Can you work these out from the model? Positions are in its coordinate system, mm. A direction names the side the tool comes from. Give positions to 0.01 mm unless a question says otherwise; leave off trailing zeros. Write each loop counter-clockwise with the first axis right and the second up, starting at its lowest first coordinate (ties: lowest second). Pieces come first, ordered by that corner, then holes.
from build123d import *

# Parameters (mm, degrees)
SKETCH_1_W      = 30
SKETCH_1_H      = 15
SKETCH_1_R      = 1.75
EXTRUDE_1_DEPTH = 1.5
FILLET_1_R      = 5
EXTRUDE_2_DEPTH = 10


with BuildPart() as part:
    # 草图1 → 凸台-拉伸1 (new body)
    with BuildSketch(Plane(origin=(0, 0, 0), x_dir=(1, 0, 0), z_dir=(0, 1, 0))):
        Rectangle(SKETCH_1_W, SKETCH_1_H)
        with Locations(Location((-8.867330988, 0, 0), (0, 0, 270))):
            Circle(SKETCH_1_R, mode=Mode.SUBTRACT)
        with Locations(Location((8.647397187, 0, 0), (0, 0, 270))):
            Circle(SKETCH_1_R, mode=Mode.SUBTRACT)
    extrude(amount=EXTRUDE_1_DEPTH)

    # 圆角1
    fillet_1_edges = [part.edges().sort_by_distance(p)[0] for p in [
        (-15, 0.75, 7.5),
        (15, 0.75, 7.5),
    ]]
    fillet(fillet_1_edges, radius=FILLET_1_R)

    # 草图2 → 凸台-拉伸2 (add)
    with BuildSketch(Plane(origin=(15, 0, 0), x_dir=(0, 0, -1), z_dir=(1, 0, 0))):
        with BuildLine():
            Line((7.5, 1.5), (7.5, 0))
            ThreePointArc((7.5, 0), (9.573370103, 7.420692388), (3.953819335, 2.149431792))
            ThreePointArc((3.953819335, 2.149431792), (4.281764154, 1.894235083), (4.689365013, 1.975072601))
            Line((4.689365013, 1.975072601), (5.099963472, 2.270889054))
            ThreePointArc((5.099963472, 2.270889054), (5.292783095, 2.555387358), (5.256408648, 2.897141058))
            ThreePointArc((5.256408648, 2.897141058), (8.821524242, 6.1221625), (7.5, 1.5))
        make_face()
    extrude_2 = extrude(amount=-EXTRUDE_2_DEPTH)

    # 镜向1: 凸台-拉伸2 across plane
    add(extrude_2.mirror(Plane(origin=(0, 0, 0), x_dir=(0, 0, 1), z_dir=(1, 0, 0))))


solid = part.part
(1) Imagine slicing it at D-D, the plane x = -6.25. Write out the boundary of the cut face in (y, z), plus the area to 3 significant figures.
Returned:
outline: (0, -7.5) arc R4 ccw (long way) to (2.15, -3.95) arc R0.5 ccw to (1.98, -4.69) - (2.27, -5.1) arc R0.5 ccw to (2.9, -5.26) arc R2.5 cw (long way) to (1.5, -7.5) - (1.5, 7.5) - (0, 7.5) - close
area: 48.4 mm2
(2) Imagine slicing it at A-A, the plane z = 0. Write out the boundary of the cut face in (x, y), plus the area to 3 significant figures.
Returned:
outline: (-15, 0) - (-10.62, 0) - (-10.62, 1.5) - (-15, 1.5) - close; (-7.12, 0) - (6.9, 0) - (6.9, 1.5) - (-7.12, 1.5) - close; (10.4, 0) - (15, 0) - (15, 1.5) - (10.4, 1.5) - close
area: 34.5 mm2
(3) Imagine slicing it at C-C, the plane z = -8.75. Write out the boundary of the cut face in (x, y), plus the area to 3 significant figures.
Returned:
outline: (-15, 0.2) - (-5, 0.2) - (-5, 1.83) - (-15, 1.83) - close; (-15, 6.17) - (-5, 6.17) - (-5, 7.8) - (-15, 7.8) - close; (5, 0.2) - (15, 0.2) - (15, 1.83) - (5, 1.83) - close; (5, 6.17) - (15, 6.17) - (15, 7.8) - (5, 7.8) - close
area: 65.4 mm2
(4) If we mould it in two halves opening along X, with no side actions, what happens to faces 1 (the face through (0, 0, 0)), 2 (the face through (0, 1, -7.5)), 3 (the face through (-15, 3, -4))? For each: +X half, -X half, draft (parallel to the pull), parting line (faces both ways), or undercut.
Returned:
face 1: draft
face 2: undercut
face 3: -X half
(5) For faces 4 (the face through (-13.57, 0.76, 6)), 5 (the face through (5, 7, -7)), 6 (the face through (0, 1.5, 0)), which set-ups out of +Z, -Z, +X, -X, +Y, -Y let a thin tool reach every point of the face, with its end or its side?
Returned:
face 4: +Z, -X, +Y, -Y
face 5: -Z, +Y
face 6: +Z, +X, -X
(6) Will these pins go through, and if not, where does the flat tip stop? P1, Ø4.5, axis at y = 4, z = -7.5, coming from the +X side; P2, Ø2, axis at x = 10.5, y = 7, coming from the +Z side; P3, Ø1.6, axis at x = -1, y = 0.5, coming from the -Z side.
Returned:
P1: passes through
P2: stops at z = -4.04
P3: stops at z = -7.5
(7) If I drill on L1, parallel to X at y = 1, z = 0; L2, parallel to Y at x = 10.5, z = -7.5; L3, parallel to Z at x = -7.5, y = 4, over which ranges is the centre line in solid material (lowest first)?
Returned:
L1: x = -15 to -10.62, -7.12 to 6.9, 10.4 to 15
L2: y = 0 to 1.5, 6.5 to 8
L3: z = -11.5 to -10, -5 to -3.5
(8) Imagine slicing it at B-B, the plane y = 5.75. Write out the boundary of the cut face in (x, z).
Returned:
outline: (-15, -11.1) - (-5, -11.1) - (-5, -9.29) - (-15, -9.29) - close; (-15, -5.71) - (-5, -5.71) - (-5, -3.9) - (-15, -3.9) - close; (5, -11.1) - (15, -11.1) - (15, -9.29) - (5, -9.29) - close; (5, -5.71) - (15, -5.71) - (15, -3.9) - (5, -3.9) - close
